Source: three-view drawing plus pictorial views. Frame: mm from the lowest corner of the part. Round coordinates to 2 decimals unless told otherwise and drop trailing zeros. Write each loop counter-clockwise with the first axis right and the second up, starting at its lowest first coordinate (ties: lowest second). Pieces come first, ordered by that corner, then holes. Notation, with made-up numbers: (37, 56.5) - (72, 56.5) arc R30 cw to (72, 89.5) - close; hole circle Ø6 at (-32.5, 67). An arc over 180 degrees is marked (long way). Write each question's results on one line, items separated by ' | '.
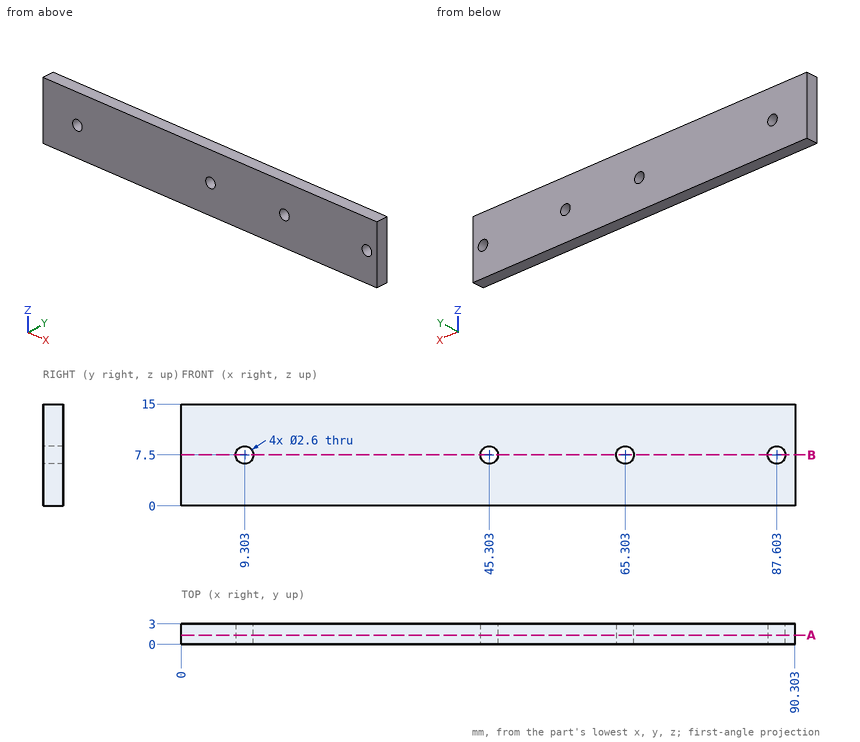
Q1. Section query B-B, the plane z = 7.5. Return loops of the section in (x, y).
Answer block:
outline: (0, 0) - (8, 0) - (8, 3) - (0, 3) - close; (10.6, 0) - (44, 0) - (44, 3) - (10.6, 3) - close; (46.6, 0) - (64, 0) - (64, 3) - (46.6, 3) - close; (66.6, 0) - (86.3, 0) - (86.3, 3) - (66.6, 3) - close; (88.9, 0) - (90.3, 0) - (90.3, 3) - (88.9, 3) - close
Q2. Ray query, line 1 along X through (y, z) = (1.1, 7.5); line 2 along Z through (x, y) = (87.5, 0.8) (1 decimal); line 3 along X through (y, z) = (2.5, 8). Return the intervals inside material, ascending.
Answer block:
line 1: 0 to 8, 10.6 to 44, 46.6 to 64, 66.6 to 86.3, 88.9 to 90.3 | line 2: 0 to 6.2, 8.8 to 15 | line 3: 0 to 8.1, 10.5 to 44.1, 46.5 to 64.1, 66.5 to 86.4, 88.8 to 90.3
Q3. Section query A-A, the plane y = 1.35. Return loops of the section in (x, z), plus the area to 3 significant figures.
Answer block:
outline: (0, 0) - (90.3, 0) - (90.3, 15) - (0, 15) - close; hole circle Ø2.6 at (9.3, 7.5); hole circle Ø2.6 at (45.3, 7.5); hole circle Ø2.6 at (65.3, 7.5); hole circle Ø2.6 at (87.6, 7.5) | area: 1,330 mm2
